Read the model definition and answer for the solid it produces. Units are mm, in the model's axes. Coordinates: 2 decimals unless noted, no trailing zeros. Write each loop counter-clockwise with the first axis right and the second up, starting at its lowest first coordinate (ties: lowest second). Pieces come first, ordered by that corner, then holes.
1) Determine the mould class of faces 1 (the face through (-19.524, 1.232, -4.336)), 2 (the face through (10.76, 1.23, -10.69)), 3 (the face through (-4, 2.5, 4)) for opening direction Z: +Z half, -Z half, draft (parallel to the pull), parting line (faces both ways), or undercut.
2) The part is cut by section C-C (y = 1.5). Determine the outline of the cut face in (x, z) (3 decimals).
3) Find the intervals of material crossed by line 1 (X direction, y = 1.65, z = 0); line 2 (Z direction, x = -10, y = 1.1) (1 decimal); line 3 (Z direction, x = -1.5, y = 0.8), in increasing order.
4) The part is cut by section B-B (x = 0). Determine the outline of the cut face in (y, z).
5) Each of these flat-tipped pins is pushed along its axis until it touches: pin 1 Ø1.5 at (y, z) = (1, -2.5) entering from -X; pin 2 Ø1.8 at (x, z) = (10, 10) entering from +Y; pin 3 Ø1.5 at (x, y) = (14.5, 0.5) entering from -Z. Where does it stop, or does it pass through?
6) The part is cut by section D-D (x = -10). Determine the outline of the cut face in (y, z) (1 decimal), then the cut area to 3 significant figures.
7) The part is cut by section A-A (z = 0). Determine the outline of the cut face in (x, y), then the cut area to 3 significant figures.
from build123d import *

# Parameters (mm, degrees)
SKETCH_1_R          = 20
SKETCH_1_R_2        = 5
EXTRUDE_1_DEPTH     = 2.5
HOLE_WIZARD_M2_51_D = 2.05


with BuildPart() as part:
    # Эскиз1 → Бобышка-Вытянуть1 (new body)
    with BuildSketch(Plane(origin=(0, 0, 0), x_dir=(1, 0, 0), z_dir=(0, 1, 0))):
        with Locations(Location((0, 0, 0), (0, 0, 270))):
            Circle(SKETCH_1_R)
        with Locations(Location((0, 0, 0), (0, 0, 270))):
            Circle(SKETCH_1_R_2, mode=Mode.SUBTRACT)
    extrude(amount=EXTRUDE_1_DEPTH)

    # Отверстие обработанное метчиком M2.51 (through all)
    with Locations(Plane(origin=(0, 2.5, 0), x_dir=(1, 0, 0), z_dir=(0, 1, 0))):
        with Locations((-10, 10), (10, 10), (10, -10), (-10, -10)):
            Hole(HOLE_WIZARD_M2_51_D / 2)


solid = part.part
Reported:
1. face 1: parting line
1. face 2: undercut
1. face 3: draft
2. outline: circle Ø40 at (0, 0); hole circle Ø2.05 at (-10, -10); hole circle Ø2.05 at (-10, 10); hole circle Ø10 at (0, 0); hole circle Ø2.05 at (10, -10); hole circle Ø2.05 at (10, 10)
3. line 1: x = -20 to -5, 5 to 20
3. line 2: z = -17.3 to -11, -9 to 9, 11 to 17.3
3. line 3: z = -19.94 to -4.77, 4.77 to 19.94
4. outline: (0, -20) - (2.5, -20) - (2.5, -5) - (0, -5) - close; (0, 5) - (2.5, 5) - (2.5, 20) - (0, 20) - close
5. pin 1: stops at x = -19.92
5. pin 2: passes through
5. pin 3: stops at z = -14.52
6. outline: (0, -17.3) - (2.5, -17.3) - (2.5, -11) - (0, -11) - close; (0, -9) - (2.5, -9) - (2.5, 9) - (0, 9) - close; (0, 11) - (2.5, 11) - (2.5, 17.3) - (0, 17.3) - close
6. area: 76.4 mm2
7. outline: (-20, 0) - (-5, 0) - (-5, 2.5) - (-20, 2.5) - close; (5, 0) - (20, 0) - (20, 2.5) - (5, 2.5) - close
7. area: 75.0 mm2
